from build123d import *

# Parameters (mm, degrees)
F0_W      = 300
F0_H      = 10
F1_DEPTH  = 300
F3_DEPTH  = 10.001
F4_SIZE   = 1
F5_R      = 2.5
F6_DEPTH  = 25
F7_SIZE   = 0.5
F8_R      = 5
F9_DEPTH  = 10.001
F10_SIZE  = 0.5
F11_R     = 4.25
F12_DEPTH = 10.001
F13_SIZE  = 0.5
F14_R     = 2.75
F15_DEPTH = 10.001


# Not quite as in the source:
# - a feature names something its author has since deleted; it is built from what else it names


with BuildPart() as f1:
    # F0 (on Right) → F1 (new body)
    with BuildSketch(Plane.YZ):
        with Locations((-150, 5)):
            Rectangle(F0_W, F0_H)
    extrude(amount=-F1_DEPTH)

    # F2 (on face) → F3 (cut, through all)
    with BuildSketch(Plane.XY.offset(10)):
        Polygon((-200, -70), (-300, -70), (-300, -110), (-200, -110), (-200, -90), align=None)
        Polygon((-200, -160), (-300, -160), (-300, -200), (-200, -200), (-200, -180), align=None)
    extrude(amount=-F3_DEPTH, mode=Mode.SUBTRACT)

    # F4
    f4_edges = [f1.edges().sort_by_distance(p)[0] for p in [
        (0, -150, 10),
        (-150, -300, 10),
        (-300, -250, 10),
        (-250, -200, 10),
        (-200, -180, 10),
        (-250, -160, 10),
        (-300, -135, 10),
        (-250, -110, 10),
        (-200, -90, 10),
        (-250, -70, 10),
        (-300, -35, 10),
        (-150, 0, 10),
        (0, -150, 0),
        (-150, 0, 0),
        (-300, -35, 0),
        (-250, -70, 0),
        (-200, -90, 0),
        (-250, -110, 0),
        (-300, -135, 0),
        (-250, -160, 0),
        (-200, -180, 0),
        (-250, -200, 0),
        (-300, -250, 0),
        (-150, -300, 0),
        (0, -300, 5),
        (0, 0, 5),
        (-300, -70, 5),
        (-200, -70, 5),
        (-200, -110, 5),
        (-300, -110, 5),
        (-300, -160, 5),
        (-200, -160, 5),
        (-200, -200, 5),
        (-300, -200, 5),
        (-300, -300, 5),
    ]]
    chamfer(f4_edges, length=F4_SIZE)

    # F5 (on face) → F6 (cut)
    with BuildSketch(Plane.XY.offset(10)):
        with Locations((-15, -50)):
            Circle(F5_R)
        with Locations((-35, -50)):
            Circle(F5_R)
        with Locations((-165, -50)):
            Circle(F5_R)
        with Locations((-185, -50)):
            Circle(F5_R)
        with Locations((-65, -135)):
            Circle(F5_R)
        with Locations((-85, -135)):
            Circle(F5_R)
        with Locations((-165, -135)):
            Circle(F5_R)
        with Locations((-185, -135)):
            Circle(F5_R)
        with Locations((-15, -227.5)):
            Circle(F5_R)
        with Locations((-35, -227.5)):
            Circle(F5_R)
        with Locations((-165, -227.5)):
            Circle(F5_R)
        with Locations((-185, -227.5)):
            Circle(F5_R)
        with Locations((-15, -142.5)):
            Circle(F5_R)
        with Locations((-35, -142.5)):
            Circle(F5_R)
        with Locations((-115, -142.5)):
            Circle(F5_R)
        with Locations((-135, -142.5)):
            Circle(F5_R)
    extrude(amount=-F6_DEPTH, mode=Mode.SUBTRACT)

    # F7
    f7_edges = [f1.edges().sort_by_distance(p)[0] for p in [
        (-17.5, -50, 10),
        (-12.5, -50, 5),
        (-17.5, -50, 0),
        (-37.5, -50, 10),
        (-32.5, -50, 5),
        (-37.5, -50, 0),
        (-167.5, -50, 10),
        (-162.5, -50, 5),
        (-167.5, -50, 0),
        (-187.5, -50, 10),
        (-182.5, -50, 5),
        (-187.5, -50, 0),
        (-67.5, -135, 10),
        (-62.5, -135, 5),
        (-67.5, -135, 0),
        (-87.5, -135, 10),
        (-82.5, -135, 5),
        (-87.5, -135, 0),
        (-187.5, -135, 10),
        (-182.5, -135, 5),
        (-187.5, -135, 0),
        (-167.5, -135, 10),
        (-162.5, -135, 5),
        (-167.5, -135, 0),
        (-17.5, -142.5, 10),
        (-12.5, -142.5, 5),
        (-17.5, -142.5, 0),
        (-37.5, -142.5, 10),
        (-32.5, -142.5, 5),
        (-37.5, -142.5, 0),
        (-117.5, -142.5, 10),
        (-112.5, -142.5, 5),
        (-117.5, -142.5, 0),
        (-137.5, -142.5, 10),
        (-132.5, -142.5, 5),
        (-137.5, -142.5, 0),
        (-17.5, -227.5, 10),
        (-12.5, -227.5, 5),
        (-17.5, -227.5, 0),
        (-37.5, -227.5, 10),
        (-32.5, -227.5, 5),
        (-37.5, -227.5, 0),
        (-167.5, -227.5, 10),
        (-162.5, -227.5, 5),
        (-167.5, -227.5, 0),
        (-187.5, -227.5, 10),
        (-182.5, -227.5, 5),
        (-187.5, -227.5, 0),
    ]]
    chamfer(f7_edges, length=F7_SIZE)

    # F8 (on face) → F9 (cut, through all)
    with BuildSketch(Plane.XY.offset(10)):
        with Locations((-284.5, -274.6)):
            Circle(F8_R)
        with Locations((-225.5, -274.6)):
            Circle(F8_R)
        with Locations((-284.5, -30)):
            Circle(F8_R)
        with Locations((-225.5, -30)):
            Circle(F8_R)
    extrude(amount=-F9_DEPTH, mode=Mode.SUBTRACT)

    # F10
    f10_edges = [f1.edges().sort_by_distance(p)[0] for p in [
        (-289.5, -30, 10),
        (-279.5, -30, 5),
        (-289.5, -30, 0),
        (-230.5, -30, 10),
        (-220.5, -30, 5),
        (-230.5, -30, 0),
        (-289.5, -274.6, 10),
        (-279.5, -274.6, 5),
        (-289.5, -274.6, 0),
        (-230.5, -274.6, 10),
        (-220.5, -274.6, 5),
        (-230.5, -274.6, 0),
    ]]
    chamfer(f10_edges, length=F10_SIZE)

    # F11 (on face) → F12 (cut, through all)
    with BuildSketch(Plane.XY.offset(10)):
        with Locations((-34, -199)):
            Circle(F11_R)
        with Locations((-160, -199)):
            Circle(F11_R)
    extrude(amount=-F12_DEPTH, mode=Mode.SUBTRACT)

    # F13
    f13_edges = [f1.edges().sort_by_distance(p)[0] for p in [
        (-164.25, -199, 10),
        (-155.75, -199, 5),
        (-164.25, -199, 0),
        (-38.25, -199, 10),
        (-29.75, -199, 5),
        (-38.25, -199, 0),
    ]]
    chamfer(f13_edges, length=F13_SIZE)

    # F14 (on face) → F15 (cut, through all)
    with BuildSketch(Plane.XY.offset(10)):
        with Locations((-193, -10)):
            Circle(F14_R)
        with Locations((-173, -10)):
            Circle(F14_R)
        with Locations((-133, -10)):
            Circle(F14_R)
        with Locations((-113, -10)):
            Circle(F14_R)
        with Locations((-73, -10)):
            Circle(F14_R)
        with Locations((-53, -10)):
            Circle(F14_R)
        with Locations((-33, -10)):
            Circle(F14_R)
    extrude(amount=-F15_DEPTH, mode=Mode.SUBTRACT)


solid = f1.part
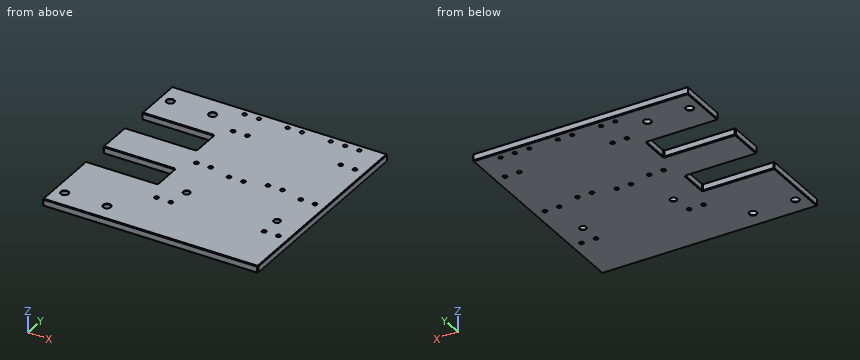
The listing builds one solid part. Answer for the finished solid, in the listing's coordinates (mm). Coordinates: 2 decimals unless noted, no trailing zeros. Order: outer loops, then holes, each group sorted by start corner. A loop starts at its lowest first (then second) coordinate and runs counter-clockwise, first axis right, second up.
Q1. A cutting plane is placed at B-B, the plane y = -30. Write down the section's boundary in (x, z), and give its area (3 significant figures).
Q2. Consider line 1 (X direction, y = -142.5, z = 2.5); line 2 (X direction, y = -227.5, z = 6); line 3 (Y direction, x = -250.5, z = 1.25). Determine where each line is inside the solid, lowest interval first.
Q3. A cutting plane is placed at D-D, the plane z = 7.25. State how many separate pieces and enclosed holes the cut face has, and give its area (3 significant figures).
Q4. A cutting plane is placed at C-C, the plane y = -186. Write down the section's boundary in (x, z), and give its area (3 significant figures).
Q5. Given P1, Ø2.5, axis at y = -186, z = 3.5, coming from the -X side, flat-ended and moving along its own axis, determine where the tip first touches the part or whether it passes through.
Q6. A cutting plane is placed at A-A, the plane x = -272. Write down the section's boundary in (y, z), and give its area (3 significant figures).
Answers follow:
1. outline: (-300, 1) - (-299, 0) - (-290, 0) - (-289.5, 0.5) - (-289.5, 9.5) - (-290, 10) - (-299, 10) - (-300, 9) - close; (-279.5, 0.5) - (-279, 0) - (-231, 0) - (-230.5, 0.5) - (-230.5, 9.5) - (-231, 10) - (-279, 10) - (-279.5, 9.5) - close; (-220.5, 0.5) - (-220, 0) - (-1, 0) - (0, 1) - (0, 9) - (-1, 10) - (-220, 10) - (-220.5, 9.5) - close
1. area: 2,800 mm2
2. line 1: x = -300 to -137.5, -132.5 to -117.5, -112.5 to -37.5, -32.5 to -17.5, -12.5 to 0
2. line 2: x = -300 to -187.5, -182.5 to -167.5, -162.5 to -37.5, -32.5 to -17.5, -12.5 to 0
2. line 3: y = -300 to -200, -160 to -110, -70 to 0
3. separate pieces: 1
3. enclosed holes: 29
3. area: 81,100 mm2
4. outline: (-200, 1) - (-199, 0) - (-1, 0) - (0, 1) - (0, 9) - (-1, 10) - (-199, 10) - (-200, 9) - close
4. area: 2,000 mm2
5. P1: stops at x = -200
6. outline: (-300, 1) - (-299, 0) - (-201, 0) - (-200, 1) - (-200, 9) - (-201, 10) - (-299, 10) - (-300, 9) - close; (-160, 1) - (-159, 0) - (-111, 0) - (-110, 1) - (-110, 9) - (-111, 10) - (-159, 10) - (-160, 9) - close; (-70, 1) - (-69, 0) - (-1, 0) - (0, 1) - (0, 9) - (-1, 10) - (-69, 10) - (-70, 9) - close
6. area: 2,190 mm2
